```python
from build123d import *

# Parameters (mm, degrees)
SKETCH_W        = 200
SKETCH_H        = 250
PAD_DEPTH       = 2.5
SKETCH001_W     = 2
SKETCH001_H     = 80
PAD001_DEPTH    = 55
SKETCH002_R     = 2.5
SKETCH002_R_2   = 6.5
POCKET_DEPTH    = 282.001
PAD002_DEPTH    = 60
POCKET001_DEPTH = 5.001


with BuildPart() as part:
    # Sketch → Pad (new body, symmetric)
    with BuildSketch(Plane.XY):
        Polygon((100, 180), (141, 180), (141, -180), (100, -180), (100, -135), (-100, -135), (-100, -180), (-141, -180), (-141, 180), (-100, 180), (-100, 135), (100, 135), align=None)
        Rectangle(SKETCH_W, SKETCH_H, mode=Mode.SUBTRACT)
    extrude(amount=PAD_DEPTH, both=True)

    # Sketch001 → Pad001 (new body)
    with BuildSketch(Plane.XY.offset(2.5)):
        with Locations((-140, 0)):
            Rectangle(SKETCH001_W, SKETCH001_H)
        with Locations((140, 0)):
            Rectangle(SKETCH001_W, SKETCH001_H)
    extrude(amount=PAD001_DEPTH)

    # Sketch002 → Pocket (cut, through all)
    with BuildSketch(Plane(origin=(-141, 0, 0), x_dir=(0, -1, 0), z_dir=(-1, 0, 0))):
        with Locations((-33.5, 30.5)):
            Circle(SKETCH002_R)
        with Locations((33.5, 30.5)):
            Circle(SKETCH002_R)
        with Locations((-0.051525, 30.52907)):
            Circle(SKETCH002_R_2)
    extrude(amount=-POCKET_DEPTH, mode=Mode.SUBTRACT)

    # Sketch003 → Pad002 (new body)
    with BuildSketch(Plane.XY.offset(2.5)):
        Polygon((-100, 98), (-103, 98), (-103, 128), (-73, 128), (-73, 125), (-100, 125), align=None)
        Polygon((73, 125), (100, 125), (100, 98), (103, 98), (103, 128), (73, 128), align=None)
        Polygon((-73, -125), (-100, -125), (-100, -98), (-103, -98), (-103, -128), (-73, -128), align=None)
        Polygon((73, -125), (100, -125), (100, -98), (103, -98), (103, -128), (73, -128), align=None)
    extrude(amount=PAD002_DEPTH)

    # Sketch004 → Pocket001 (cut, through all)
    with BuildSketch(Plane.XY.offset(2.5)):
        Polygon((-100, 180), (-154.538937, 125.461063), (-154.538937, 180), align=None)
        Polygon((100, 180), (154.538937, 125.461063), (154.538937, 180), align=None)
        Polygon((-100, -180), (-154.538937, -125.461063), (-154.538937, -180), align=None)
        Polygon((100, -180), (154.538937, -125.461063), (154.538937, -180), align=None)
    extrude(amount=-POCKET001_DEPTH, mode=Mode.SUBTRACT)


solid = part.part
```
Model file for the job. Use its own axes, mm. A direction names the side the tool comes from. Coordinates: 2 decimals unless noted, no trailing zeros. Loops run counter-clockwise (first coordinate to the right, second up) from the corner with the lowest first, then second, coordinate; pieces in that order, holes last. Notation, with made-up numbers: (63, 40.25) - (121, 40.25) arc R12 ccw to (121, 63.25) - close; hole circle Ø7 at (-30.75, -16). An arc over 180 degrees is marked (long way). Answer as a JSON object with one key per item and string values. Group by question number.
(1) Cut at D-D (x = 17.5). Give the cut face in (y, z).
(2) Tool access for faces 1 (the face through (-103, -113, 32)), 2 (the face through (103, -113, 32)), 3 (the face through (88, 128, 32)), 4 (the face through (100, -1, 1)): list every direction of +Z, -Z, +X, -X, +Y, -Y with a clear straight run to the whole face (end or side of a thin tool).
(3) Cut at A-A (y = 17). Give the cut face in (x, z), then the cut area to 3 significant figures.
(4) Probe line 1 along Y through (x, z) = (140, 30); line 2 along X through (y, z) = (-126, 17.5); line 3 along X through (y, z) = (-34, 2). List the from-to ranges inside material, lowest first.
(5) Flat gauge pins, fed straight in: pin 1 (15 mm diameter, centred on x = 83, z = 33, fed in from +Y); pin 2 (10 mm diameter, centred on x = 44, y = 117.5, fed in from +Z); pin 3 (1 mm diameter, centred on x = 139.5, y = -14.5, fed in from +Z); pin 4 (10 mm diameter, centred on y = -114, z = 50.5, fed in from -X). Where does each tip first touch, or does it go through?
(6) Two-plate mould, pull along Y, no slides. Class faces 5 (the face through (-100, 1, -1)), 6 (the face through (-88, 128, 32)), 7 (the face through (141, 2, 21)): released by +Y, released by -Y, zero draft, split by the parting line, or undercut.
(7) Cut at C-C (z = 52). State how many separate pieces and enclosed holes the cut face has, then the cut area to 3 significant figures.
(8) Cut at B-B (x = -85.5). Give the cut face in (y, z), then the cut area to 3 significant figures.
Geometry says:
{
 "1": {"outline": "(-135, -2.5) - (-125, -2.5) - (-125, 2.5) - (-135, 2.5) - close; (125, -2.5) - (135, -2.5) - (135, 2.5) - (125, 2.5) - close"},
 "2": {"face 1": "+Z, -X, +Y, -Y", "face 2": "+Z, +X, +Y, -Y", "face 3": "+Z, +X, -X, +Y", "face 4": "+Z, -Z"},
 "3": {"outline": "(-141, -2.5) - (-100, -2.5) - (-100, 2.5) - (-139, 2.5) - (-139, 57.5) - (-141, 57.5) - close; (100, -2.5) - (141, -2.5) - (141, 57.5) - (139, 57.5) - (139, 2.5) - (100, 2.5) - close", "area": "630 mm^2"},
 "4": {"line 1": "y = -40 to -35.95, -31.05 to -6.43, 6.53 to 31.05, 35.95 to 40", "line 2": "x = -103 to -73, 73 to 103", "line 3": "x = -141 to -100, 100 to 141"},
 "5": {"pin 1": "stops at y = 128", "pin 2": "passes through", "pin 3": "stops at z = 57.5", "pin 4": "stops at x = -103"},
 "6": {"face 5": "undercut", "face 6": "released by +Y", "face 7": "zero draft"},
 "7": {"separate pieces": "6", "enclosed holes": "0", "area": "1,000 mm^2"},
 "8": {"outline": "(-135, -2.5) - (-125, -2.5) - (-125, 62.5) - (-128, 62.5) - (-128, 2.5) - (-135, 2.5) - close; (125, -2.5) - (135, -2.5) - (135, 2.5) - (128, 2.5) - (128, 62.5) - (125, 62.5) - close", "area": "460 mm^2"}
}
